```python
from build123d import *

# Parameters (mm, degrees)
BOSS_EXTRUDE1_DEPTH      = 50
BOSS_EXTRUDE2_DEPTH      = 10
BOSS_EXTRUDE2_DEPTH_BACK = 23
SKETCH3_R                = 25
CUT_EXTRUDE1_REACH       = 173.917
SKETCH6_R                = 13
CUT_EXTRUDE2_DEPTH       = 174.304008792


with BuildPart() as part:
    # Sketch1 → Boss-Extrude1 (new body)
    with BuildSketch(Plane.XY):
        Polygon((0, 6.5), (0, 0), (47.634193477, 0), (114.765880418, 56.330173752), (110.587760955, 61.309462632), (45.268386955, 6.5), align=None)
        Polygon((47.634193477, 0), (0, 0), (0, -6.5), (50, -6.5), (118.943999881, 51.350884872), (114.765880418, 56.330173752), align=None)
    extrude(amount=BOSS_EXTRUDE1_DEPTH)

    # Sketch3 → Boss-Extrude2 (add, two sides: drawn at the far end of the back side and taken through both)
    with BuildSketch(Plane(origin=(15.50318183, -18.475972642, 0), x_dir=(0.7660444431189771, 0.6427876096865404, 0), z_dir=(-0.6427876096865404, 0.7660444431189771, 0)).offset(-BOSS_EXTRUDE2_DEPTH_BACK)):
        with Locations(Location((124.124102693, -25, 0), (0, 0, 180))):
            Circle(SKETCH3_R)
    extrude(amount=BOSS_EXTRUDE2_DEPTH + BOSS_EXTRUDE2_DEPTH_BACK)

    # Sketch5 → Cut-Extrude1 (cut, up to next)
    with BuildSketch(Plane(origin=(0, 6.5, 0), x_dir=(1, 0, 0), z_dir=(0, 1, 0)), mode=Mode.PRIVATE) as cut_extrude1_sk1:
        with BuildLine():
            Line((0, -13), (20, -13))
            ThreePointArc((20, -13), (32, -25), (20, -37))
            Line((20, -37), (0, -37))
            ThreePointArc((0, -37), (-12, -25), (0, -13))
        make_face()
    cut_extrude1_tool1 = extrude(cut_extrude1_sk1.sketch, amount=-CUT_EXTRUDE1_REACH, mode=Mode.PRIVATE) & part.part
    add(cut_extrude1_tool1.solids().sort_by_distance((10, 6.5, 25))[0], mode=Mode.SUBTRACT)

    # Sketch6 → Cut-Extrude2 (cut, through all)
    with BuildSketch(Plane(origin=(9.075305733, -10.815528211, 0), x_dir=(0.7660444431189771, 0.6427876096865404, 0), z_dir=(-0.6427876096865404, 0.7660444431189771, 0))):
        with Locations(Location((124.124102693, -25, 0), (0, 0, 180))):
            Circle(SKETCH6_R)
    extrude(amount=-CUT_EXTRUDE2_DEPTH, mode=Mode.SUBTRACT)


solid = part.part
```
Check sheet for the modelled part. Datum: model origin and axes. Units: mm. A direction names the side the tool comes from. Round coordinates to 2 decimals unless told otherwise and drop trailing zeros. Loops run counter-clockwise (first coordinate to the right, second up) from the corner with the lowest first, then second, coordinate; pieces in that order, holes last. Notation, with made-up numbers: (-38, 87) - (-31, 87) arc R32 ccw to (-31, 119) - close; hole circle Ø1 at (75.25, -27). An arc over 180 degrees is marked (long way). Answer as a JSON object with one key per item and string values. Group by question number.
Q1. Sectioned sample at C-C, the plane x = 35. Enter the section's corners in (y, z), plus the area to 3 significant figures.
Q2. Sectioned sample at D-D, the plane z = 4. Enter the section's corners in (x, y), plus the area to 3 significant figures.
Q3. Sectioned sample at A-A, the plane x = 17.5. Enter the section's corners in (y, z), plus the area to 3 significant figures.
Q4. Gauge pin test, flat ends, axial feed: P1, Ø8, axis at y = 72, z = 19, coming from the +X side; P2, Ø6, axis at x = 74.5, z = 18, coming from the +Y side; P3, Ø1.5, axis at x = 72, z = 13.5, coming from the +Y side. Record the tip position at first contact, or that the pin passes through.
Q5. Set-up check for faces 5 (the face through (33, 6.5, 25)), 6 (the face through (36, -6.5, 25)), 7 (the face through (10, 0, 37)): record each of +Z, -Z, +X, -X, +Y, -Y from which the full face is reachable in a straight line by a thin tool's end or side.
Q6. Sectioned sample at B-B, the plane z = 25. Enter the section's corners in (x, y).
Q7. Scan lines: line 1 along Y through (x, z) = (26, 48); line 2 along X through (y, z) = (40, 5); line 3 along Y through (x, z) = (93, 43). Record each from-to range of solid material in increasing order. Write a range as [from, to].
Q8. Mould release check, pull along X, two halves, no side actions. Record for faces 1 (the face through (134.047, 72.207, 26.099)), 2 (the face through (32, 0, 25)), 3 (the face through (117.128, 36.773, 14.239)), 4 (the face through (121.957, 62.666, 33.786)): released by +X, released by -X, zero draft, split by the parting line, or undercut.
Solution:
{
 "1": {"outline": "(-6.5, 0) - (6.5, 0) - (6.5, 50) - (-6.5, 50) - close", "area": "650 mm²"},
 "2": {"outline": "(0, -6.5) - (50, -6.5) - (108.55, 42.63) - (114.98, 34.97) - (135.76, 52.41) - (114.55, 77.69) - (93.77, 60.25) - (100.2, 52.59) - (45.27, 6.5) - (0, 6.5) - close", "area": "2,480 mm²"},
 "3": {"outline": "(-6.5, 0) - (6.5, 0) - (6.5, 13) - (-6.5, 13) - close; (-6.5, 37) - (6.5, 37) - (6.5, 50) - (-6.5, 50) - close", "area": "338 mm²"},
 "4": {"P1": "stops at x = 136.85", "P2": "stops at y = 33.55", "P3": "stops at y = 29.56"},
 "5": {"face 5": "+Z, -Z, -X, +Y", "face 6": "+Z, -Z, +X, -X, -Y", "face 7": "-X, +Y, -Y"},
 "6": {"outline": "(32, -6.5) - (50, -6.5) - (99.79, 35.28) - (106.22, 27.62) - (115.41, 35.33) - (94.2, 60.61) - (85.01, 52.9) - (91.44, 45.24) - (45.27, 6.5) - (32, 6.5) - close; (114.12, 77.33) - (135.33, 52.05) - (144.52, 59.76) - (123.31, 85.04) - close"},
 "7": {"line 1": "y = [-6.5, 6.5]", "line 2": "x = [85.19, 105.42], [108.89, 120.97]", "line 3": "y = [29.58, 46.55], [55.28, 59.61]"},
 "8": {"face 1": "undercut", "face 2": "released by -X", "face 3": "released by +X", "face 4": "undercut"}
}
